Build history of the part. All positions in model axes, mm. A direction names the side the tool comes from. Round coordinates to 2 decimals unless told otherwise and drop trailing zeros. Write each loop counter-clockwise with the first axis right and the second up, starting at its lowest first coordinate (ties: lowest second). Pieces come first, ordered by that corner, then holes.
Item 1: Drop flat-ended pins along their axis: pin 1 Ø7.5 at (x, z) = (0, 0) entering from -Y; pin 2 Ø6 at (y, z) = (-101.5, 0.5) entering from -X; pin 3 Ø1.5 at (y, z) = (116.5, 1.5) entering from -X. Give the stop position or say it passes through.
Item 2: 3-axis set-ups, long thin cutter, end or side, ignore diameter. For faces 1 (the flat face through (5.474, 2.8, 3.219)), 2 (the cylindrical face through (2.93, -189.86, 1.22)): which of +Z, -Z, +X, -X, +Y, -Y reach the whole face in a straight line?
Item 3: Mould opens along Z. For faces 3 (the flat face through (2, -200, -3)), 4 (the cylindrical face through (2.52, 189.86, 1.93)), 5 (the flat face through (0, 3, -6.35)) say: +Z half, -Z half, draft (parallel to the pull), parting line (faces both ways), or undercut.
Item 4: Wall check: probe 1 along Y at (x, z) = (-4.75, 2.75); probe 2 along Y at (x, z) = (-4.5, 3.25); probe 3 along Z at (x, y) = (0, 189.75) (3 decimals). Give the ranges that are in metal, low to high.
Item 5: Band-saw the part on A-A, the plane y = 34.5. Write the cut outline in (x, z).
```python
from build123d import *

# Parameters (mm, degrees)
BOSS_EXTRUDE1_DEPTH             = 200
F_1_4_0_25_DIAMETER_HOLE1_D     = 6.35
F_1_4_0_25_DIAMETER_HOLE1_DEPTH = 20
F_1_4_0_25_DIAMETER_HOLE1_TIP   = 1.907732465
F_1_4_0_25_DIAMETER_HOLE2_D     = 6.35
F_1_4_0_25_DIAMETER_HOLE2_DEPTH = 20
F_1_4_0_25_DIAMETER_HOLE2_TIP   = 1.907732465
M6X1_0_TAPPED_HOLE3_REACH       = 202.537
M6X1_0_TAPPED_HOLE3_BORE_R      = 2.5
M6X1_0_TAPPED_HOLE4_REACH       = 202.637
M6X1_0_TAPPED_HOLE4_BORE_R      = 2.5


with BuildPart() as part:
    # Sketch1 → Boss-Extrude1 (new, symmetric)
    with BuildSketch(Plane(origin=(0, 0, 0), x_dir=(1, 0, 0), z_dir=(0, 1, 0))):
        Polygon((7.332348419, 0), (3.666174209, 6.35), (-3.666174209, 6.35), (-7.332348419, 0), (-3.666174209, -6.35), (3.666174209, -6.35), align=None)
    extrude(amount=BOSS_EXTRUDE1_DEPTH, both=True)

    # 1_4 _0.25_ Diameter Hole1
    with Locations(Plane(origin=(0, 200, 0), x_dir=(1, 0, 0), z_dir=(0, 1, 0))):
        with Locations((0, 0)):
            Hole(F_1_4_0_25_DIAMETER_HOLE1_D / 2, depth=F_1_4_0_25_DIAMETER_HOLE1_DEPTH)
            with Locations((0, 0, -(F_1_4_0_25_DIAMETER_HOLE1_DEPTH + F_1_4_0_25_DIAMETER_HOLE1_TIP / 2))):  # 118° drill point
                Cone(0, F_1_4_0_25_DIAMETER_HOLE1_D / 2, F_1_4_0_25_DIAMETER_HOLE1_TIP, mode=Mode.SUBTRACT)

    # 1_4 _0.25_ Diameter Hole2
    with Locations(Plane(origin=(0, -200, 0), x_dir=(-1, 0, 0), z_dir=(0, -1, 0))):
        with Locations((0, 0)):
            Hole(F_1_4_0_25_DIAMETER_HOLE2_D / 2, depth=F_1_4_0_25_DIAMETER_HOLE2_DEPTH)
            with Locations((0, 0, -(F_1_4_0_25_DIAMETER_HOLE2_DEPTH + F_1_4_0_25_DIAMETER_HOLE2_TIP / 2))):  # 118° drill point
                Cone(0, F_1_4_0_25_DIAMETER_HOLE2_D / 2, F_1_4_0_25_DIAMETER_HOLE2_TIP, mode=Mode.SUBTRACT)

    # M6x1.0 Tapped Hole3 bore → M6x1.0 Tapped Hole3 (cut, up to next)
    with BuildSketch(Plane(origin=(0, 0, -6.35), x_dir=(-1, 0, 0), z_dir=(0, 0, -1)), mode=Mode.PRIVATE) as m6x1_0_tapped_hole3_sk1:
        with Locations((0, -194)):
            Circle(M6X1_0_TAPPED_HOLE3_BORE_R)
    m6x1_0_tapped_hole3_tool1 = extrude(m6x1_0_tapped_hole3_sk1.sketch, amount=-M6X1_0_TAPPED_HOLE3_REACH, mode=Mode.PRIVATE) & part.part
    # M6x1.0 Tapped Hole3 bore → M6x1.0 Tapped Hole3 (cut, up to next)
    with BuildSketch(Plane(origin=(0, 0, -6.35), x_dir=(-1, 0, 0), z_dir=(0, 0, -1)), mode=Mode.PRIVATE) as m6x1_0_tapped_hole3_sk2:
        with Locations((0, 194)):
            Circle(M6X1_0_TAPPED_HOLE3_BORE_R)
    m6x1_0_tapped_hole3_tool2 = extrude(m6x1_0_tapped_hole3_sk2.sketch, amount=-M6X1_0_TAPPED_HOLE3_REACH, mode=Mode.PRIVATE) & part.part
    add(m6x1_0_tapped_hole3_tool1.solids().sort_by_distance((0, -194, -6.35))[0], mode=Mode.SUBTRACT)
    add(m6x1_0_tapped_hole3_tool2.solids().sort_by_distance((0, 194, -6.35))[0], mode=Mode.SUBTRACT)

    # M6x1.0 Tapped Hole4 bore → M6x1.0 Tapped Hole4 (cut, up to next)
    with BuildSketch(Plane(origin=(-5.499261314, 0, 3.175), x_dir=(-0.5000000000000001, 0, -0.8660254037844386), z_dir=(-0.8660254037844386, 0, 0.5000000000000001)), mode=Mode.PRIVATE) as m6x1_0_tapped_hole4_sk1:
        with Locations((0, -194)):
            Circle(M6X1_0_TAPPED_HOLE4_BORE_R)
    m6x1_0_tapped_hole4_tool1 = extrude(m6x1_0_tapped_hole4_sk1.sketch, amount=-M6X1_0_TAPPED_HOLE4_REACH, mode=Mode.PRIVATE) & part.part
    # M6x1.0 Tapped Hole4 bore → M6x1.0 Tapped Hole4 (cut, up to next)
    with BuildSketch(Plane(origin=(-5.499261314, 0, 3.175), x_dir=(-0.5000000000000001, 0, -0.8660254037844386), z_dir=(-0.8660254037844386, 0, 0.5000000000000001)), mode=Mode.PRIVATE) as m6x1_0_tapped_hole4_sk2:
        with Locations((0, 194)):
            Circle(M6X1_0_TAPPED_HOLE4_BORE_R)
    m6x1_0_tapped_hole4_tool2 = extrude(m6x1_0_tapped_hole4_sk2.sketch, amount=-M6X1_0_TAPPED_HOLE4_REACH, mode=Mode.PRIVATE) & part.part
    add(m6x1_0_tapped_hole4_tool1.solids().sort_by_distance((-5.499261, 194, 3.175))[0], mode=Mode.SUBTRACT)
    add(m6x1_0_tapped_hole4_tool2.solids().sort_by_distance((-5.499261, -194, 3.175))[0], mode=Mode.SUBTRACT)


solid = part.part
```
Results:
1. pin 1: stops at y = -200
1. pin 2: stops at x = -7.33
1. pin 3: stops at x = -6.9
2. face 1: +Z, +X, +Y, -Y
2. face 2: -Y
3. face 3: draft
3. face 4: undercut
3. face 5: -Z half
4. probe 1: y = -200 to -196.5, -191.5 to 191.5, 196.5 to 200
4. probe 2: y = -200 to -196.44, -191.56 to 191.56, 196.44 to 200
4. probe 3: z = -6.35 to -3.175, 3.175 to 6.35
5. outline: (-7.33, 0) - (-3.67, -6.35) - (3.67, -6.35) - (7.33, 0) - (3.67, 6.35) - (-3.67, 6.35) - close
